CAD build for the part. Positions are in the model's coordinates, mm. A direction names the side the tool comes from. Round coordinates to 2 decimals unless told otherwise and drop trailing zeros. Order: outer loops, then holes, each group sorted by start corner. A loop starts at its lowest first (then second) coordinate and runs counter-clockwise, first axis right, second up. Notation, with made-up numbers: M -12.75,23 L 25.25,23 A13 cw 25.25,45 Z; hole C 4.5,-35.5 d11. An arc over 180 degrees is marked long. Answer as a JSON object with one key per item and string values. Group by question number.
```python
from build123d import *

# Parameters (mm, degrees)
SKETCH_W     = 60
SKETCH_H     = 30
SKETCH_R     = 2.25
SKETCH_R_2   = 2.05
PAD_DEPTH    = 5.5
SKETCH001_W  = 75
SKETCH001_H  = 45
POCKET_DEPTH = 5.501


with BuildPart() as part:
    # Sketch → Pad (new body)
    with BuildSketch(Plane.XY):
        Rectangle(SKETCH_W, SKETCH_H)
        with Locations((25, 0)):
            Circle(SKETCH_R, mode=Mode.SUBTRACT)
        with Locations((-25, 0)):
            Circle(SKETCH_R, mode=Mode.SUBTRACT)
        Circle(SKETCH_R_2, mode=Mode.SUBTRACT)
    extrude(amount=PAD_DEPTH)

    # Sketch001 → Pocket (cut, through all)
    with BuildSketch(Plane.XY.offset(5.5)):
        Rectangle(SKETCH001_W, SKETCH001_H)
        with BuildLine():
            ThreePointArc((-27, 9.5), (-24.525126, 10.525126), (-23.5, 13))
            Line((-23.5, 13), (-23.5, 18))
            Line((-23.5, 18), (-3.5, 18))
            Line((-3.5, 18), (-3.5, 13))
            ThreePointArc((-3.5, 13), (0, 9.5), (3.5, 13))
            Line((3.5, 13), (3.5, 18))
            Line((3.5, 18), (23.5, 18))
            Line((23.5, 18), (23.5, 13))
            ThreePointArc((23.5, 13), (24.525126, 10.525127), (26.999998, 9.5))
            Line((26.999998, 9.5), (31.999998, 9.5))
            Line((31.999998, 9.5), (31.999998, -9.5))
            Line((31.999998, -9.5), (26.999998, -9.5))
            ThreePointArc((26.999998, -9.5), (24.525126, -10.525127), (23.5, -13))
            Line((23.5, -13), (23.5, -18))
            Line((23.5, -18), (6, -18))
            Line((6, 0), (6, -18))
            ThreePointArc((6, 0), (0, 6), (-6, 0))
            Line((-6, 0), (-6, -18))
            Line((-23.5, -18), (-6, -18))
            Line((-23.5, -18), (-23.5, -13))
            ThreePointArc((-23.5, -13), (-24.525126, -10.525127), (-27, -9.5))
            Line((-27, -9.5), (-32, -9.5))
            Line((-32, -9.5), (-32, 9.5))
            Line((-32, 9.5), (-27, 9.5))
        make_face(mode=Mode.SUBTRACT)
    extrude(amount=-POCKET_DEPTH, mode=Mode.SUBTRACT)


solid = part.part
```
Item 1: 3-axis set-ups, long thin cutter, end or side, ignore diameter. For faces 1 (the face through (23.5, 14, 3)), 2 (the face through (-6, -7, 3)), 3 (the face through (-3.5, 14, 3)): which of +Z, -Z, +X, -X, +Y, -Y reach the whole face in a straight line?
Item 2: Flat gauge pins, fed straight in: pin 1 Ø1.5 at (x, z) = (29, 2) entering from -Y; pin 2 Ø1.6 at (y, z) = (13.5, 4) entering from +X; pin 3 Ø0.6 at (y, z) = (14, 3.5) entering from -X; pin 4 Ø6 at (x, y) = (-21.5, -1) entering from -Z. Where does each tip first touch, or does it go through?
Item 3: Cut at D-D, the plane x = 0. Give the cut face in (y, z), and give its area (4 significant figures).
Item 4: Two-plate mould, pull along X, no slides. Class faces 4 (the face through (27.146, 0.676, 2.712)), 5 (the face through (-24.55, 10.5, 2.79)), 6 (the face through (-29, 9.5, 3)): +X half, -X half, draft (parallel to the pull), parting line (faces both ways), or undercut.
Item 5: Cut at A-A, the plane y = -6. Give the cut face in (x, z), and give its area (3 significant figures).
Item 6: Cut at B-B, the plane x = -25. Give the cut face in (y, z).
Item 7: Drill centre lines: line 1 (X direction, y = -4.25, z = 0.95); line 2 (Y direction, x = -25, z = 2.6); line 3 (X direction, y = 12, z = 1.75). Where is each one in solid material? Low to high. Write a range as [from, to].
Item 8: Cut at C-C, the plane z = 3.75. Give the cut face in (x, y), and give its area (3 significant figures).
Response values:
{
 "1": {"face 1": "+Z, -Z, +X, +Y", "face 2": "+Z, -Z, -Y", "face 3": "+Z, -Z, +Y"},
 "2": {"pin 1": "y = -9.5", "pin 2": "x = 23.51", "pin 3": "x = -23.5", "pin 4": "z = 0"},
 "3": {"outline": "M 6,0 L 9.5,0 L 9.5,5.5 L 6,5.5 Z", "area": "19.25 mm^2"},
 "4": {"face 4": "undercut", "face 5": "-X half", "face 6": "draft"},
 "5": {"outline": "M -30,0 L -6,0 L -6,5.5 L -30,5.5 Z; M 6,0 L 30,0 L 30,5.5 L 6,5.5 Z", "area": "264 mm^2"},
 "6": {"outline": "M -10.13,0 L -2.25,0 L -2.25,5.5 L -10.13,5.5 Z; M 2.25,0 L 10.13,0 L 10.13,5.5 L 2.25,5.5 Z"},
 "7": {"line 1": "[-30, -6], [6, 30]", "line 2": "[-10.13, -2.25], [2.25, 10.13]", "line 3": "[-23.65, -3.35], [3.35, 23.65]"},
 "8": {"outline": "M -30,-9.5 L -27,-9.5 A3.5 cw -23.5,-13 L -23.5,-15 L -6,-15 L -6,0 A6 cw 6,0 L 6,-15 L 23.5,-15 L 23.5,-13 A3.5 cw 27,-9.5 L 30,-9.5 L 30,9.5 L 27,9.5 A3.5 cw 23.5,13 L 23.5,15 L 3.5,15 L 3.5,13 A3.5 cw -3.5,13 L -3.5,15 L -23.5,15 L -23.5,13 A3.5 cw -27,9.5 L -30,9.5 Z; hole C -25,0 d4.5; hole C 25,0 d4.5", "area": "1,370 mm^2"}
}
